```python
from build123d import *

# Parameters (mm, degrees)
CYLINDER026_R     = 2
CYLINDER026_DEPTH = 5
CYLINDER_R        = 1.6
CYLINDER_DEPTH    = 5
BOX001_W          = 10
BOX001_H          = 10
BOX001_DEPTH      = 10
BOX_W             = 15
BOX_H             = 10
BOX_DEPTH         = 10
CYLINDER025_R     = 4
CYLINDER025_DEPTH = 43


with BuildPart() as cylinder001:
    # Cylinder026 → Cylinder026 (new body)
    with BuildSketch(Plane(origin=(0, 0, 0), x_dir=(0, 0, -1), z_dir=(1, 0, 0))):
        Circle(CYLINDER026_R)
    extrude(amount=CYLINDER026_DEPTH)


with BuildPart() as cylinder:
    # Cylinder → Cylinder (new body)
    with BuildSketch(Plane(origin=(38, -4, 0), x_dir=(1, 0, 0), z_dir=(0, 1, 0))):
        Circle(CYLINDER_R)
    extrude(amount=CYLINDER_DEPTH)


with BuildPart() as cube001:
    # Box001 → Box001 (new body)
    with BuildSketch(Plane(origin=(33, -13, -5), x_dir=(1, 0, 0), z_dir=(0, 0, 1))):
        with Locations((5, 5)):
            Rectangle(BOX001_W, BOX001_H)
    extrude(amount=BOX001_DEPTH)


with BuildPart() as cube:
    # Box → Box (new body)
    with BuildSketch(Plane(origin=(28, 0, -5), x_dir=(1, 0, 0), z_dir=(0, 0, 1))):
        with Locations((7.5, 5)):
            Rectangle(BOX_W, BOX_H)
    extrude(amount=BOX_DEPTH)


with BuildPart() as piston:
    # Cylinder025 → Cylinder025 (new body)
    with BuildSketch(Plane.ZY.offset(-43)):
        Circle(CYLINDER025_R)
    extrude(amount=CYLINDER025_DEPTH)

    # Cut: cut Cube
    add(cube.part, mode=Mode.SUBTRACT)

    # Cut001: cut Cube001
    add(cube001.part, mode=Mode.SUBTRACT)

    # Cut002: cut Cylinder
    add(cylinder.part, mode=Mode.SUBTRACT)

    # Cut003: cut Cylinder001
    add(cylinder001.part, mode=Mode.SUBTRACT)


solid = piston.part
```
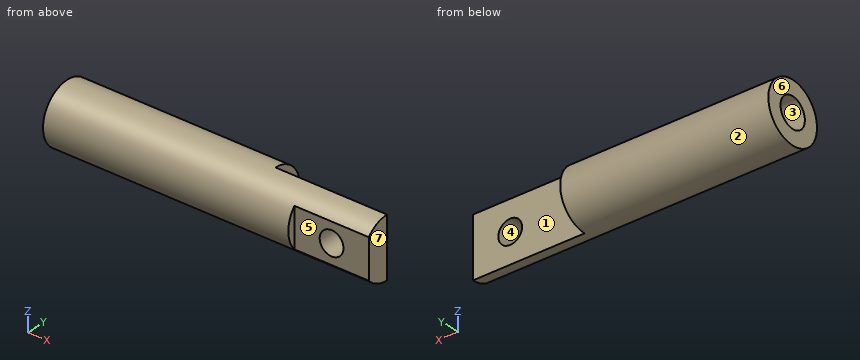
Here's how the part is built. I have some questions about the finished solid (model axes, mm). Face numbers are marked on the shaded views. A direction names the side the tool comes from. Give positions to 0.01 mm unless a question says otherwise; leave off trailing zeros. Write each loop counter-clockwise with the first axis right and the second up, starting at its lowest first coordinate (ties: lowest second). Pieces come first, ordered by that corner, then holes. Notation, with made-up numbers: (25.25, 14.25) -> (37.25, 14.25) arc R21 cw to (37.25, 18.25) -> close; hole circle Ø2 at (-24.75, 44). An arc over 180 degrees is marked (long way). Write each question's results on one line, items separated by ' | '.
Item 1: Suppose I cut it at D-D on x = 9. Write out the boundary of the cut face in (y, z).
Output:
outline: circle Ø8 at (0, 0)
Item 2: If I drill on L1, parallel to Y at x = 1.35, z = 0; L2, parallel to X at y = 2.75, z = 2.75; L3, parallel to Z at x = 38, y = -1.4, over which ranges is the centre line in solid material (lowest first)?
Output:
L1: y = -4 to -2, 2 to 4 | L2: x = 0 to 28 | L3: z = -3.75 to -1.6, 1.6 to 3.75
Item 3: We'd pull the mould along X, two halves only. Please class the marked faces 4, 5, 6 and 7: pulls with the +X half, pulls with the -X half, needs draft (parallel to the pull), parting line crosses it, or undercut.
Output:
face 4: undercut | face 5: needs draft | face 6: pulls with the -X half | face 7: pulls with the +X half
Item 4: For pin 1 Ø1 at (y, z) = (1.5, 0.5) entering from -X; pin 2 Ø1.6 at (x, z) = (35.5, 1) entering from -Y; pin 3 Ø3.5 at (x, z) = (38, 0) entering from +Y; pin 4 Ø0.5 at (y, z) = (-3.5, 0) entering from +X, each with a flat end and sliding along its axis, tell me the tip position at first contact or that it passes through.
Output:
pin 1: stops at x = 0 | pin 2: stops at y = -3 | pin 3: stops at y = 0 | pin 4: stops at x = 33
Item 5: Suppose I cut it at B-B on z = 0. Write out the boundary of the cut face in (x, y).
Output:
outline: (0, -4) -> (33, -4) -> (33, -3) -> (36.4, -3) -> (36.4, 0) -> (28, 0) -> (28, 4) -> (0, 4) -> (0, 2) -> (5, 2) -> (5, -2) -> (0, -2) -> close; (39.6, -3) -> (43, -3) -> (43, 0) -> (39.6, 0) -> close
Item 6: On a 3-axis mill with a long thin cutter (end or side, diameter ignored), from which of +Z, -Z, +X, -X, +Y, -Y can I reach the whole of each face in a straight line? I mean the marked faces 1, 2 and 3. Say none if no direction works.
Output:
face 1: +Z, -Z, +X, +Y | face 2: +X, -X | face 3: -X
Item 7: Suppose I cut it at A-A on x = 38. Write out the boundary of the cut face in (y, z), plus the area to 3 significant figures.
Output:
outline: (-3, -2.65) arc R4 ccw to (0, -4) -> (0, -1.6) -> (-3, -1.6) -> close; (-3, 1.6) -> (0, 1.6) -> (0, 4) arc R4 ccw to (-3, 2.65) -> close | area: 11.9 mm^2
Item 8: Suppose I cut it at C-C on y = 0.75. Write out the boundary of the cut face in (x, z).
Output:
outline: (0, -3.93) -> (28, -3.93) -> (28, 3.93) -> (0, 3.93) -> (0, 1.85) -> (5, 1.85) -> (5, -1.85) -> (0, -1.85) -> close
